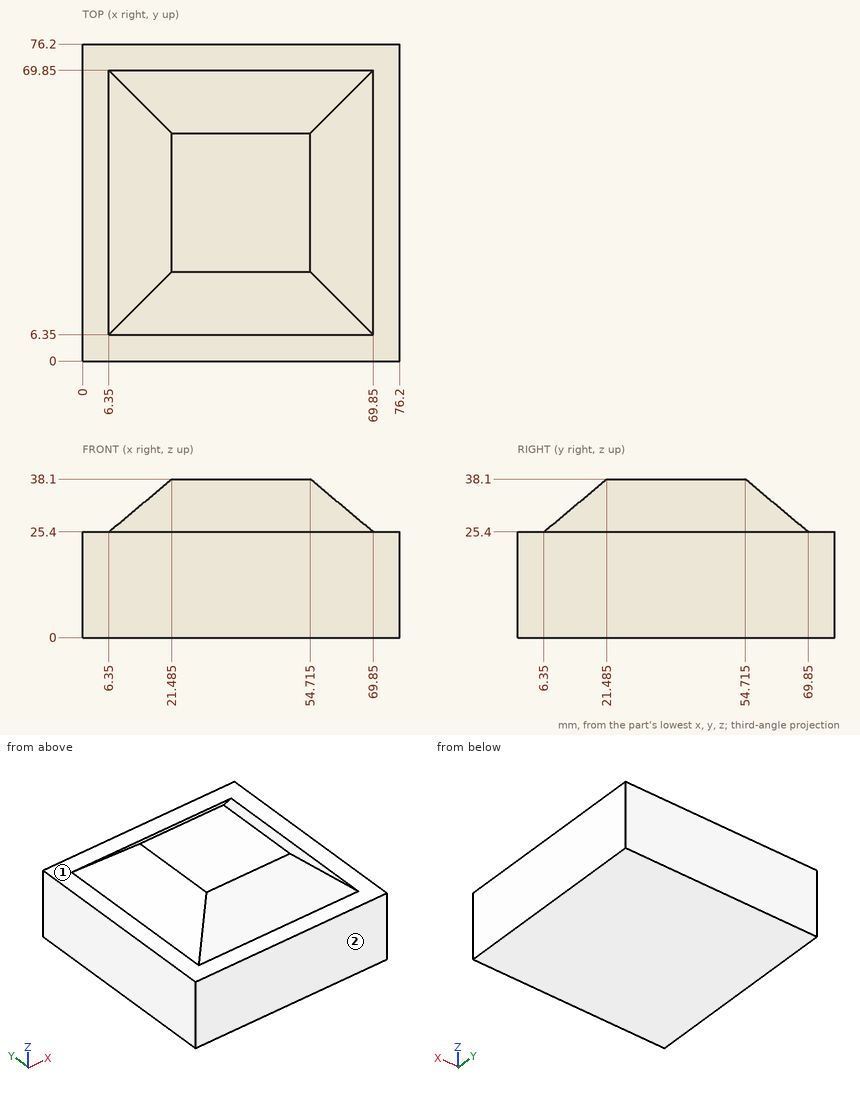
The drawing under review shows one solid part. Ordinate dimensions are in mm from its lowest x, y, z. A direction names the side the tool comes from. Coordinates: 2 decimals unless noted, no trailing zeros.
1) Machinability: for the marked faces 1 and 2, which of the approach directions +Z, -Z, +X, -X, +Y, -Y give a long, thin tool a straight path to every point of the face, cutting with its end or side? Answer none if there is none.
2) To check wall thickness, follow L1, parallel to Z at x = 72.5, y = 50; L2, parallel to Y at x = 31.5, z = 35.5 (1 decimal); L3, parallel to Z at x = 26.5, y = 13. State the ranges of each line that lie inside material, in increasing order.
3) Insertion check: pin 1 (8 mm diameter, centred on y = 13, z = 31.5, fed in from -X); pin 2 (6 mm diameter, centred on y = 54, z = 30, fed in from +X). Each pin has a flat end and moves straight along its axis. Give the tip position at first contact, or say it passes through.
Check result:
1. face 1: +Z
1. face 2: +Z, -Z, +X, -X, -Y
2. L1: z = 0 to 25.4
2. L2: y = 18.4 to 57.8
2. L3: z = 0 to 30.98
3. pin 1: stops at x = 8.85
3. pin 2: stops at x = 67.94
